```python
from build123d import *

# Parameters (mm, degrees)
BOSS_EXTRUDE1_DEPTH = 1.5
BOSS_EXTRUDE2_DEPTH = 7
SKETCH5_R           = 1.5875
CUT_EXTRUDE1_DEPTH  = 1.5


with BuildPart() as part:
    # Sketch1 → Boss-Extrude1 (new body)
    with BuildSketch(Plane.XY):
        Polygon((-2.742413779, 4.75), (-5.484827557, 0), (-2.742413779, -4.75), (2.742413779, -4.75), (4.568284005, -1.5875), (14.755382296, -1.5875), (14.755382296, -9.179038244), (-14.755382296, -9.179038244), (-14.755382296, 9.179038244), (14.755382296, 9.179038244), (14.755382296, 1.5875), (4.568284005, 1.5875), (2.742413779, 4.75), align=None)
    extrude(amount=BOSS_EXTRUDE1_DEPTH)

    # Sketch4 → Boss-Extrude2 (add)
    with BuildSketch(Plane(origin=(0, 0, 0), x_dir=(-1, 0, 0), z_dir=(0, 0, -1))):
        with BuildLine():
            Line((-4.568284005, 1.5875), (-2.545553722, 1.5875))
            ThreePointArc((-2.545553722, 1.5875), (3, 0), (-2.545553722, -1.5875))
            Line((-2.545553722, -1.5875), (-4.568284005, -1.5875))
            Line((-4.568284005, -1.5875), (-14.755382296, -1.5875))
            Line((-14.755382296, -1.5875), (-14.755382296, -9.179038244))
            Line((-14.755382296, -9.179038244), (14.755382296, -9.179038244))
            Line((14.755382296, -9.179038244), (14.755382296, 9.179038244))
            Line((14.755382296, 9.179038244), (-14.755382296, 9.179038244))
            Line((-14.755382296, 9.179038244), (-14.755382296, 1.5875))
            Line((-14.755382296, 1.5875), (-4.568284005, 1.5875))
        make_face()
    extrude(amount=BOSS_EXTRUDE2_DEPTH)

    # Sketch5 → Cut-Extrude1 (cut)
    with BuildSketch(Plane.XY.offset(1.5)):
        with Locations((3.200685555, 5.54375)):
            Circle(SKETCH5_R)
        with Locations((6.40137111, 0)):
            Circle(SKETCH5_R)
        with Locations((3.200685555, -5.54375)):
            Circle(SKETCH5_R)
        with Locations((-3.200685555, -5.54375)):
            Circle(SKETCH5_R)
        with Locations((-6.40137111, 0)):
            Circle(SKETCH5_R)
        with Locations((-3.200685555, 5.54375)):
            Circle(SKETCH5_R)
    extrude(amount=-CUT_EXTRUDE1_DEPTH, mode=Mode.SUBTRACT)


solid = part.part
```
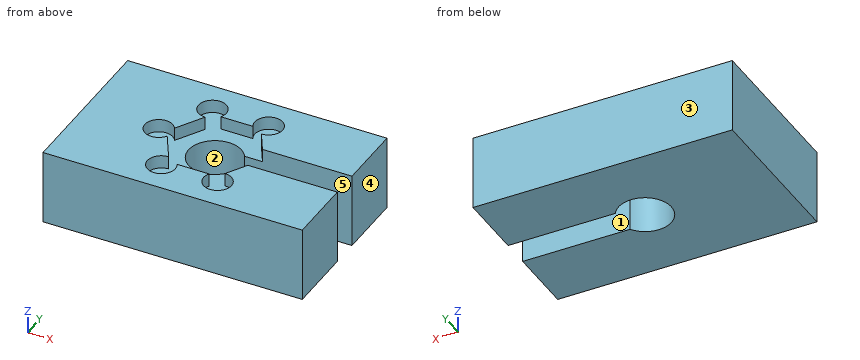
Work out the finished part from the listing and answer in its coordinate system (mm). Face numbers are marked on the shaded views. A direction names the side the tool comes from. Round coordinates to 2 decimals unless told otherwise and drop trailing zeros. Write each loop counter-clockwise with the first axis right and the second up, starting at its lowest first coordinate (ties: lowest second). Pieces come first, ordered by that corner, then holes. Notation, with made-up numbers: (22, 21.25) - (41, 21.25) arc R19 cw to (41, 46.25) - close; hole circle Ø6 at (73.25, -20.75). An arc over 180 degrees is marked (long way). Return JSON: item names as keys, results as strings. Group by question number.
Q1. Find the intervals of material crossed by L1, parallel to Y at x = 3.25, z = -3; L2, parallel to X at y = 5.5, z = 0.75; L3, parallel to Y at x = 0, z = -5.5, in increasing order.
Q2. The part is cut by section C-C on x = 7. Write down the section's boundary in (y, z), then the cut area to 3 significant figures.
Q3. The part is cut by section D-D on y = 0. Write down the section's boundary in (x, z).
Q4. This flat-tipped pin is pushed along its axis until it touches: pin 1 Ø3 at (x, y) = (-3.2, 5.54) entering from +Z. Where does it stop, or does it pass through?
Q5. For the marked faces 1 and 2, determine the directions among +Z, -Z, +X, -X, +Y, -Y from which every point of the face is accessible in a straight line to the end or side of a thin tool.
Q6. The part is cut by section A-A on x = 0. Write down the section's boundary in (y, z), then the cut area to 3 significant figures.
Q7. The part is cut by section B-B on z = -4. Write down the section's boundary in (x, y), then the cut area to 3 significant figures.
Q8. The mould has two halves that part along Y. Classify the marked faces 3, 4 and 5: released by +Y, released by -Y, zero draft, split by the parting line, or undercut.
Solved:
{
 "1": {"L1": "-9.18 to -1.59, 1.59 to 9.18", "L2": "-14.76 to -4.79, -1.61 to 1.61, 4.79 to 14.76", "L3": "-9.18 to -3, 3 to 9.18"},
 "2": {"outline": "(-9.18, -7) - (-1.59, -7) - (-1.59, 1.5) - (-9.18, 1.5) - close; (1.59, -7) - (9.18, -7) - (9.18, 1.5) - (1.59, 1.5) - close", "area": "129 mm²"},
 "3": {"outline": "(-14.76, -7) - (-3, -7) - (-3, 0) - (-7.99, 0) - (-7.99, 1.5) - (-14.76, 1.5) - close"},
 "4": {"pin 1": "z = 0"},
 "5": {"face 1": "+Z, -Z, +X", "face 2": "+Z, -Z"},
 "6": {"outline": "(-9.18, -7) - (-3, -7) - (-3, 0) - (-4.75, 0) - (-4.75, 1.5) - (-9.18, 1.5) - close; (3, -7) - (9.18, -7) - (9.18, 1.5) - (4.75, 1.5) - (4.75, 0) - (3, 0) - close", "area": "99.8 mm²"},
 "7": {"outline": "(-14.76, -9.18) - (14.76, -9.18) - (14.76, -1.59) - (2.55, -1.59) arc R3 cw (long way) to (2.55, 1.59) - (14.76, 1.59) - (14.76, 9.18) - (-14.76, 9.18) - close", "area": "476 mm²"},
 "8": {"face 3": "released by +Y", "face 4": "zero draft", "face 5": "undercut"}
}
